Answer from the drawing. Dimensions are ordinates in mm from the lowest x, y and z of the part. A direction names the side the tool comes from. Coordinates: 2 decimals unless noted, no trailing zeros. Write each loop counter-clockwise with the first axis right and the second up, starting at its lowest first coordinate (ties: lowest second). Pieces come first, ordered by that corner, then holes. Notation, with made-up numbers: (19.5, 9) - (23.5, 9) arc R21 cw to (23.5, 40) - close; hole circle Ø11 at (-22, 65.5). An arc over 180 degrees is marked (long way). Answer as a JSON object with one key per item and string values. Group by question number.
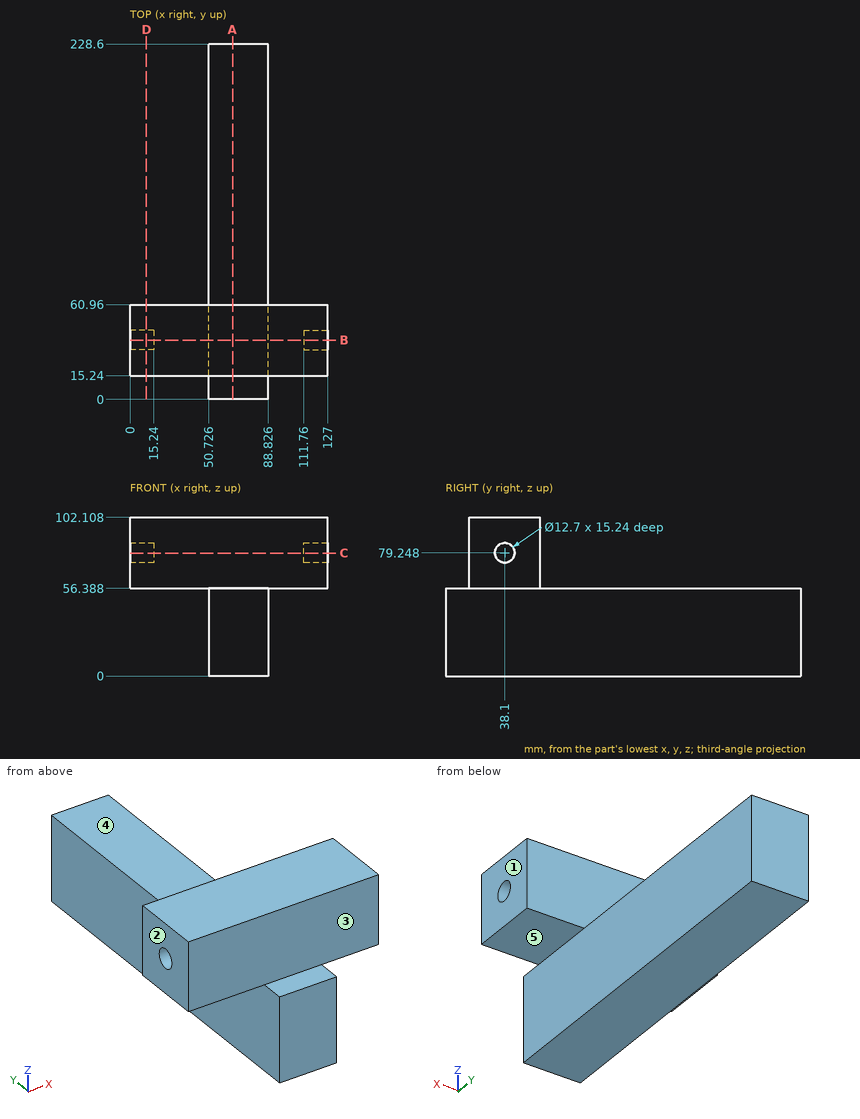
Q1. Section D-D on x = 10.5 is taken. Determine the outline of the cut face in (y, z).
Q2. Section B-B on y = 38.1 is taken. Determine the outline of the cut face in (x, z).
Q3. Flat-ended cylindrical pins translate along their axes: pin 1 Ø8 at (y, z) = (39.5, 50) entering from -X; pin 2 Ø6.5 at (y, z) = (37, 80) entering from +X; pin 3 Ø23 at (x, z) = (66, 84.5) entering from +Y. Find the tip coordinate at first contact, or state that the pin passes through.
Q4. Consider L1, parallel to Z at x = 3, y = 38; L2, parallel to Y at x = 69, z = 84; L3, parallel to X at y = 125, z = 15. Determine where each line is inside the solid, lowest interval first. Write a range as from..to.
Q5. Section A-A on x = 66 is taken. Determine the outline of the cut face in (y, z).
Q6. Section C-C on z = 79 is taken. Determine the outline of the cut face in (x, y) (3 decimals), plus the area to 3 significant figures.
Q7. A tool of negligible diameter and unlimited length cuts with its end or side. For the marked faces 1, 2, 3, 4 and 5, from which of +Z, -Z, +X, -X, +Y, -Y can it reach the whole face along a straight path? Write none if from no direction.
Numbers:
{
 "1": {"outline": "(15.24, 56.39) - (60.96, 56.39) - (60.96, 102.11) - (15.24, 102.11) - close; hole circle Ø12.7 at (38.1, 79.25)"},
 "2": {"outline": "(0, 56.39) - (50.73, 56.39) - (50.73, 0) - (88.83, 0) - (88.83, 56.39) - (127, 56.39) - (127, 72.9) - (111.76, 72.9) - (111.76, 85.6) - (127, 85.6) - (127, 102.11) - (0, 102.11) - (0, 85.6) - (15.24, 85.6) - (15.24, 72.9) - (0, 72.9) - close"},
 "3": {"pin 1": "stops at x = 50.73", "pin 2": "stops at x = 111.76", "pin 3": "stops at y = 60.96"},
 "4": {"L1": "z = 56.39..72.9, 85.6..102.11", "L2": "y = 15.24..60.96", "L3": "x = 50.73..88.83"},
 "5": {"outline": "(0, 0) - (228.6, 0) - (228.6, 56.39) - (60.96, 56.39) - (60.96, 102.11) - (15.24, 102.11) - (15.24, 56.39) - (0, 56.39) - close"},
 "6": {"outline": "(0, 15.24) - (127, 15.24) - (127, 31.755) - (111.76, 31.755) - (111.76, 44.445) - (127, 44.445) - (127, 60.96) - (0, 60.96) - (0, 44.445) - (15.24, 44.445) - (15.24, 31.755) - (0, 31.755) - close", "area": "5,420 mm²"},
 "7": {"face 1": "+Z, -Z, +X, +Y, -Y", "face 2": "+Z, -Z, -X, +Y, -Y", "face 3": "+Z, +X, -X, -Y", "face 4": "+Z, +X, -X, +Y", "face 5": "-Z, +X, +Y, -Y"}
}
